For this review, take the finished solid that the model builds, in its own axes (mm). Face numbers are marked on the shaded views. A direction names the side the tool comes from. Give positions to 0.01 mm unless a question says otherwise; leave off trailing zeros. Loops run counter-clockwise (first coordinate to the right, second up) from the corner with the lowest first, then second, coordinate; pieces in that order, holes last. Notation, with made-up numbers: (63.25, 14.25) - (89.25, 14.25) arc R22 ccw to (89.25, 38.25) - close; hole circle Ø7 at (42.25, 72). An arc over 180 degrees is marked (long way). Put each result on its own line as item: value.
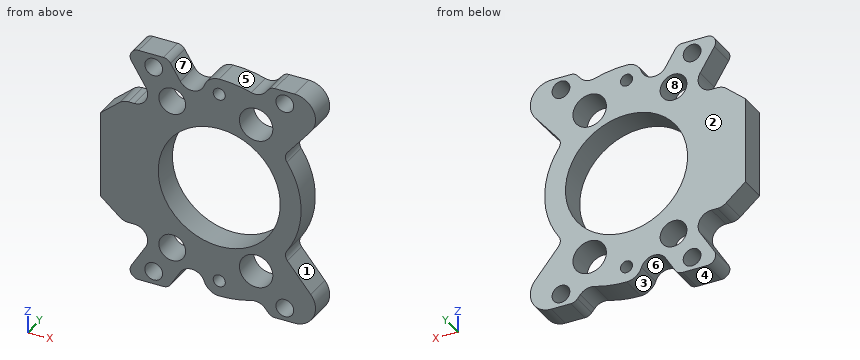
from build123d import *

# Parameters (mm, degrees)
SKETCH1_W           = 56.515
SKETCH1_H           = 56.515
SKETCH1_R           = 2.1082
SKETCH1_R_2         = 14.5
BOSS_EXTRUDE1_DEPTH = 6.35
SKETCH3_R           = 1.435
SKETCH3_R_2         = 3.96875
SKETCH3_R_3         = 3.175
CUT_EXTRUDE1_DEPTH  = 81.176137036
FILLET1_R           = 2


with BuildPart() as part:
    # Sketch1 → Boss-Extrude1 (new body)
    with BuildSketch(Plane(origin=(0, 0, 0), x_dir=(1, 0, 0), z_dir=(0, 1, 0))):
        with Locations((28.2575, 28.2575)):
            Rectangle(SKETCH1_W, SKETCH1_H)
        with Locations(Location((43.8277, 3.0607, 0), (0, 0, 270))):
            Circle(SKETCH1_R, mode=Mode.SUBTRACT)
        with Locations(Location((12.6873, 3.0607, 0), (0, 0, 270))):
            Circle(SKETCH1_R, mode=Mode.SUBTRACT)
        with Locations(Location((12.6873, 53.4543, 0), (0, 0, 270))):
            Circle(SKETCH1_R, mode=Mode.SUBTRACT)
        with Locations(Location((43.8277, 53.4543, 0), (0, 0, 270))):
            Circle(SKETCH1_R, mode=Mode.SUBTRACT)
        with Locations(Location((28.2575, 28.2575, 0), (0, 0, 270))):
            Circle(SKETCH1_R_2, mode=Mode.SUBTRACT)
    extrude(amount=BOSS_EXTRUDE1_DEPTH)

    # Sketch3 → Cut-Extrude1 (cut, through all)
    with BuildSketch(Plane(origin=(0, 6.35, 0), x_dir=(1, 0, 0), z_dir=(0, 1, 0))):
        with BuildLine():
            Line((16.085813501, 0), (40.518749208, 0))
            Line((40.518749208, 0), (39.213305633, 1.585036242))
            ThreePointArc((39.213305633, 1.585036242), (37.691149508, 2.60271564), (35.860147574, 2.610623974))
            ThreePointArc((35.860147574, 2.610623974), (32.098630453, 1.784717433), (28.2575, 1.5075))
            ThreePointArc((28.2575, 1.5075), (26.074260862, 2.211458651), (24.713448522, 4.058153181))
            ThreePointArc((24.713448522, 4.058153181), (22.067676274, 6.203891014), (19.001857165, 4.718948313))
            Line((19.001857165, 4.718948313), (16.085813501, 0))
        make_face()
        with BuildLine():
            ThreePointArc((49.976496805, 8.178709811), (50.638799533, 2.866171171), (46.116988554, 0))
            Line((46.116988554, 0), (56.515, 0))
            Line((56.515, 0), (56.515, 56.515))
            Line((56.515, 56.515), (46.116988554, 56.515))
            ThreePointArc((46.116988554, 56.515), (50.638799533, 53.648828829), (49.976496805, 48.336290189))
            Line((49.976496805, 48.336290189), (44.431541374, 41.603746953))
            ThreePointArc((44.431541374, 41.603746953), (43.977403924, 40.422997575), (44.322647522, 39.20594508))
            ThreePointArc((44.322647522, 39.20594508), (47.698626885, 28.2575), (44.322647522, 17.30905492))
            ThreePointArc((44.322647522, 17.30905492), (43.977403924, 16.092002425), (44.431541374, 14.911253047))
            Line((44.431541374, 14.911253047), (49.976496805, 8.178709811))
        make_face()
        with BuildLine():
            Line((0, 0), (5.506106862, 0))
            Line((5.506106862, 0), (10.776226353, 8.52848048))
            ThreePointArc((10.776226353, 8.52848048), (10.848364266, 11.743703095), (8.0753008, 13.3725))
            Line((8.0753008, 13.3725), (6.662712379, 13.3725))
            ThreePointArc((6.662712379, 13.3725), (5.569380258, 13.566686374), (4.609786847, 14.125492205))
            Line((4.609786847, 14.125492205), (0, 18.032807917))
            Line((0, 18.032807917), (0, 0))
        make_face()
        with BuildLine():
            Line((39.213305633, 54.929963758), (40.518749208, 56.515))
            Line((40.518749208, 56.515), (16.085813501, 56.515))
            Line((16.085813501, 56.515), (19.001857165, 51.796051687))
            ThreePointArc((19.001857165, 51.796051687), (22.067676274, 50.311108986), (24.713448522, 52.456846819))
            ThreePointArc((24.713448522, 52.456846819), (26.074260862, 54.303541349), (28.2575, 55.0075))
            ThreePointArc((28.2575, 55.0075), (32.098630453, 54.730282567), (35.860147574, 53.904376026))
            ThreePointArc((35.860147574, 53.904376026), (37.691149508, 53.91228436), (39.213305633, 54.929963758))
        make_face()
        with BuildLine():
            Line((10.776226353, 47.98651952), (5.506106862, 56.515))
            Line((5.506106862, 56.515), (0, 56.515))
            Line((0, 56.515), (0, 38.482192083))
            Line((0, 38.482192083), (4.609786847, 42.389507795))
            ThreePointArc((4.609786847, 42.389507795), (5.569380258, 42.948313626), (6.662712379, 43.1425))
            Line((6.662712379, 43.1425), (8.0753008, 43.1425))
            ThreePointArc((8.0753008, 43.1425), (10.848364266, 44.771296905), (10.776226353, 47.98651952))
        make_face()
        with Locations(Location((28.2575, 51.27, 0), (0, 0, 270))):
            Circle(SKETCH3_R)
        with Locations(Location((28.2575, 5.245, 0), (0, 0, 270))):
            Circle(SKETCH3_R)
        with Locations(Location((37.008353254, 10.1975, 0), (0, 0, 270))):
            Circle(SKETCH3_R_2)
        with Locations(Location((17.097439516, 10.1975, 0), (0, 0, 270))):
            Circle(SKETCH3_R_3)
        with Locations(Location((17.097439516, 46.3175, 0), (0, 0, 270))):
            Circle(SKETCH3_R_3)
        with Locations(Location((37.008353254, 46.3175, 0), (0, 0, 270))):
            Circle(SKETCH3_R_2)
    extrude(amount=-CUT_EXTRUDE1_DEPTH, mode=Mode.SUBTRACT)

    # Fillet1
    fillet1_edges = [part.edges().sort_by_distance(p)[0] for p in [
        (40.518749208, 3.175, 0),
        (16.085813501, 3.175, 0),
        (5.506106862, 3.175, 0),
        (5.506106862, 3.175, -56.515),
        (16.085813501, 3.175, -56.515),
        (40.518749208, 3.175, -56.515),
    ]]
    fillet(fillet1_edges, radius=FILLET1_R)


solid = part.part
1) Take a section at C-C on y = 4.5. State how many separate pieces and enclosed holes the cut face has, and give its area (3 significant figures).
Geometry check:
separate pieces: 1
enclosed holes: 11
area: 1,380 mm²
2) Insertion check: pin 1 Ø1.5 at (x, z) = (41.5, -29) entering from +Y; pin 2 Ø2 at (x, y) = (40, 1) entering from -Z; pin 3 Ø0.7 at (x, y) = (7, 1.5) entering from -Z. Each pin has a flat end and moves straight along its axis. Give the tip position at first contact, or say it passes through.
Geometry check:
pin 1: passes through
pin 2: stops at z = -56.46
pin 3: stops at z = -55.5
3) For the marked faces 1, 2, 3, 4 and 5, list the 3-axis set-ups (+Z, -Z, +X, -X, +Y, -Y) from which the entire face can be reached by the end or side of a thin tool; tool diameter is ignored.
Geometry check:
face 1: +X, +Y, -Y
face 2: +Z, -Z, +X, -X, +Y
face 3: -Z, +Y, -Y
face 4: -Z, +X, -X, +Y, -Y
face 5: +Z, +Y, -Y
4) Take a section at B-B on x = 25.5. State the section outline as (y, z) points, and give its area (3 significant figures).
Geometry check:
outline: (0, -53.79) - (6.35, -53.79) - (6.35, -42.49) - (0, -42.49) - close; (0, -14.02) - (6.35, -14.02) - (6.35, -2.72) - (0, -2.72) - close
area: 144 mm²
5) Wall thickness on line 1 (X direction, y = 4, z = -9); line 2 (Z direction, x = 36, y = 1); line 3 (Z direction, x = 46, y = 3.25) (3 decimals): over which ranges is each line inside the solid? List them lowest first.
Geometry check:
line 1: x = 11.02 to 14.16, 20.04 to 33.22, 40.79 to 49.3
line 2: z = -53.87 to -50.16, -42.48 to -40.52, -16 to -14.04, -6.36 to -2.65
line 3: z = -56.515 to -43.508, -36.205 to -20.31, -13.007 to 0
6) Take a section at A-A on z = -20.5. State the section outline as (x, y) points, and give its area (3 significant figures).
Geometry check:
outline: (0, 0) - (16.01, 0) - (16.01, 6.35) - (0, 6.35) - close; (40.51, 0) - (46.08, 0) - (46.08, 6.35) - (40.51, 6.35) - close
area: 137 mm²
7) Draft analysis for pull direction Z (two halves, no side actions). For the marked faces 6, 7 and 8, state which applies: pulls with the +Z half, pulls with the -Z half, needs draft (parallel to the pull), parting line crosses it, or undercut.
Geometry check:
face 6: pulls with the -Z half
face 7: pulls with the +Z half
face 8: undercut
